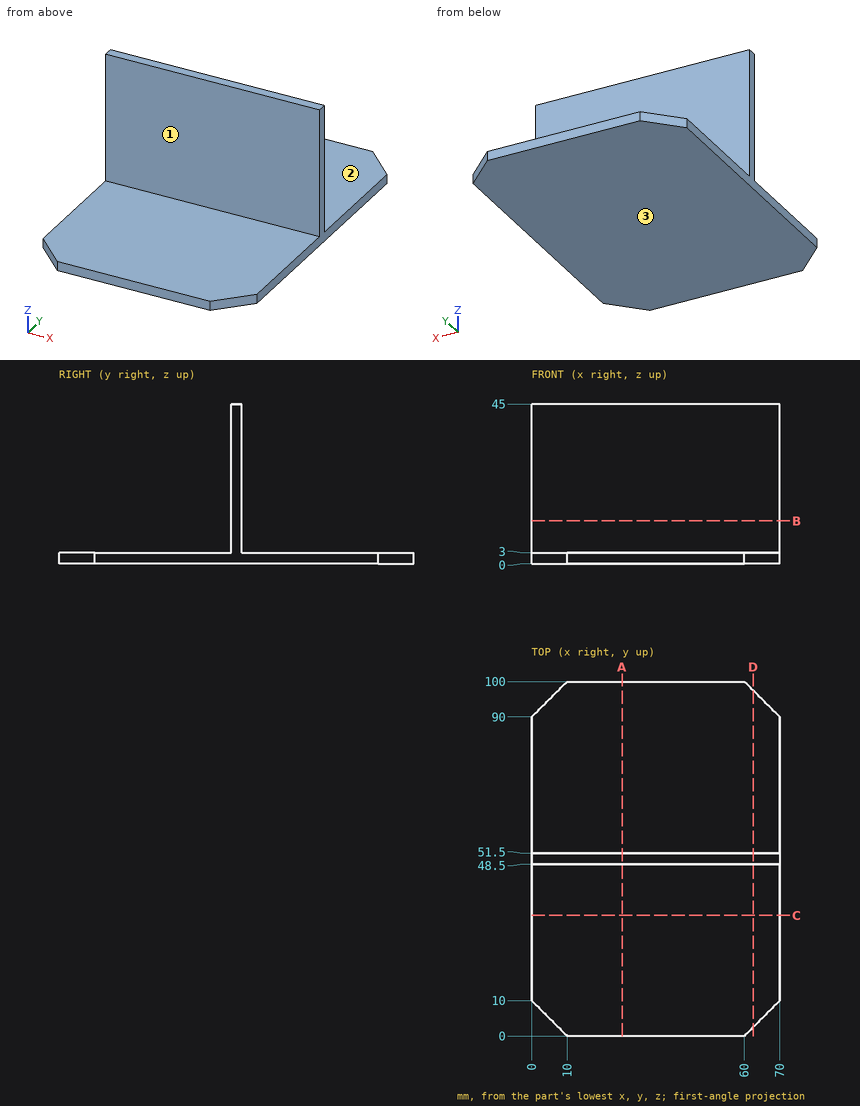
Input: dimensioned drawing with shaded views. Units: mm. Origin: part minimum x, y, z. A direction names the side the tool comes from. Round coordinates to 2 decimals unless told otherwise and drop trailing zeros. Order: outer loops, then holes, each group sorted by start corner. A loop starts at its lowest first (then second) coordinate and runs counter-clockwise, first axis right, second up.
1. Set-up query: the marked faces 1, 2 and 3. Return all of +Z, -Z, +X, -X, +Y, -Y with unobstructed straight access to the full face (end or side cutting, diameter ignored); none if empty.
The answers:
face 1: +Z, +X, -X, -Y
face 2: +Z, +X, -X, +Y
face 3: -Z, +X, -X, +Y, -Y
2. Pin query (flat end, axial travel): P1, Ø6, axis at x = 36.5, y = 82.5, coming from the +Z side; P2, Ø10, axis at x = 25, z = 26, coming from the -Y side; P3, Ø4, axis at x = 19.5, z = 8.5, coming from the +Y side. Return the tip coordinate at first contact, or that it passes through.
The answers:
P1: stops at z = 3
P2: stops at y = 48.5
P3: stops at y = 51.5
3. Cut plane B-B, the plane z = 12. Output: boundary loops of the cut face in (x, y).
The answers:
outline: (0, 48.5) - (70, 48.5) - (70, 51.5) - (0, 51.5) - close
4. Cut plane D-D, the plane x = 62.5. Output: boundary loops of the cut face in (y, z), then the cut area to 3 significant figures.
The answers:
outline: (2.5, 0) - (97.5, 0) - (97.5, 3) - (51.5, 3) - (51.5, 45) - (48.5, 45) - (48.5, 3) - (2.5, 3) - close
area: 411 mm2
5. Cut plane C-C, the plane y = 34. Output: boundary loops of the cut face in (x, z).
The answers:
outline: (0, 0) - (70, 0) - (70, 3) - (0, 3) - close
6. Cut plane A-A, the plane x = 25.5. Output: boundary loops of the cut face in (y, z).
The answers:
outline: (0, 0) - (100, 0) - (100, 3) - (51.5, 3) - (51.5, 45) - (48.5, 45) - (48.5, 3) - (0, 3) - close
7. Material intervals for line 1 (Z direction, x = 29, y = 54); line 2 (Y direction, x = 32, z = 15.5), sorted ascending.
The answers:
line 1: z = 0 to 3
line 2: y = 48.5 to 51.5
